```python
from build123d import *

# Parameters (mm, degrees)
SKETCH_W   = 140
SKETCH_H   = 140
SKETCH_W_2 = 50
SKETCH_H_2 = 50
PAD_DEPTH  = 261


with BuildPart() as part:
    # Sketch → Pad (new body)
    with BuildSketch(Plane.YZ):
        Rectangle(SKETCH_W, SKETCH_H)
        with Locations((-35.003519, 35)):
            Rectangle(SKETCH_W_2, SKETCH_H_2, mode=Mode.SUBTRACT)
        with Locations((35.282258, 35)):
            Rectangle(SKETCH_W_2, SKETCH_H_2, mode=Mode.SUBTRACT)
        with Locations((-35, -35)):
            Rectangle(SKETCH_W_2, SKETCH_H_2, mode=Mode.SUBTRACT)
        with Locations((35, -35)):
            Rectangle(SKETCH_W_2, SKETCH_H_2, mode=Mode.SUBTRACT)
    extrude(amount=PAD_DEPTH)


solid = part.part
```
Check sheet for the modelled part. Datum: model origin and axes. Units: mm. A direction names the side the tool comes from. Round coordinates to 2 decimals unless told otherwise and drop trailing zeros. Loops run counter-clockwise (first coordinate to the right, second up) from the corner with the lowest first, then second, coordinate; pieces in that order, holes last. Notation, with made-up numbers: (-39.75, -30) -> (9.25, -30) arc R33 ccw to (9.25, 7) -> close; hole circle Ø9 at (-18, -21.5). An arc over 180 degrees is marked (long way). Write item = value, one per line. Start each with the question number.
1) Thickness scan on probe 1 along Z at (x, y) = (219.5, -59.5); probe 2 along Y at (x, z) = (102, 18). Record the ranges inside material, lowest first.
2) Sectioned sample at A-A, the plane y = -43.5. Record the cut outline in (x, z).
3) Sectioned sample at B-B, the plane x = 161.5. Record the cut outline in (y, z), plus the area to 3 significant figures.
4) Sectioned sample at C-C, the plane z = 50.5. Record the cut outline in (x, y), plus the area to 3 significant figures.
5) Release check for a two-part mould opening along Y. For faces 1 (the flat face through (129, 35, 60)), 2 (the flat face through (129, -10, -35)), 3 (the flat face through (261, -1, 1)), 4 (the flat face through (129, -70, -1)) record: released by +Y, released by -Y, zero draft, split by the parting line, or undercut.
6) Set-up check for faces 5 (the flat face through (0, -1, 1)), 6 (the flat face through (129, -35, -60)): record each of +Z, -Z, +X, -X, +Y, -Y from which the full face is reachable in a straight line by a thin tool's end or side.
Results are:
q1.probe_1 = -70 to -60, -10 to 10, 60 to 70
q1.probe_2 = -70 to -60, -10 to 10.28, 60.28 to 70
q2.outline = (0, -70) -> (261, -70) -> (261, -60) -> (0, -60) -> close; (0, -10) -> (261, -10) -> (261, 10) -> (0, 10) -> close; (0, 60) -> (261, 60) -> (261, 70) -> (0, 70) -> close
q3.outline = (-70, -70) -> (70, -70) -> (70, 70) -> (-70, 70) -> close; hole (-60, -60) -> (-10, -60) -> (-10, -10) -> (-60, -10) -> close; hole (-60, 10) -> (-10, 10) -> (-10, 60) -> (-60, 60) -> close; hole (10, -60) -> (60, -60) -> (60, -10) -> (10, -10) -> close; hole (10.28, 10) -> (60.28, 10) -> (60.28, 60) -> (10.28, 60) -> close
q3.area = 9,600 mm^2
q4.outline = (0, -70) -> (261, -70) -> (261, -60) -> (0, -60) -> close; (0, -10) -> (261, -10) -> (261, 10.28) -> (0, 10.28) -> close; (0, 60.28) -> (261, 60.28) -> (261, 70) -> (0, 70) -> close
q4.area = 10,400 mm^2
q5.face_1 = undercut
q5.face_2 = undercut
q5.face_3 = zero draft
q5.face_4 = released by -Y
q6.face_5 = +Z, -Z, -X, +Y, -Y
q6.face_6 = +X, -X
